CAD build for the part. Positions are in the model's coordinates, mm. A direction names the side the tool comes from. Round coordinates to 2 decimals unless told otherwise and drop trailing zeros. Order: outer loops, then holes, each group sorted by start corner. A loop starts at its lowest first (then second) coordinate and runs counter-clockwise, first axis right, second up. Notation, with made-up numbers: (31.25, 2.25) - (84.25, 2.25) arc R10 cw to (84.25, 6.25) - close; hole circle Ø11 at (23.25, 88.25). An arc over 180 degrees is marked (long way). Write item = value, one per line.
from build123d import *

# Parameters (mm, degrees)
CYLINDER291_R     = 2
CYLINDER291_DEPTH = 10
CYLINDER290_R     = 2
CYLINDER290_DEPTH = 10
BOX400_W          = 33
BOX400_H          = 22
BOX400_DEPTH      = 5
BOX397_W          = 33
BOX397_H          = 4
BOX397_DEPTH      = 20


with BuildPart() as cylinder291:
    # Cylinder291 → Cylinder291 (new body)
    with BuildSketch(Plane(origin=(-15, 72, 32), x_dir=(1, 0, 0), z_dir=(0, 0, 1))):
        Circle(CYLINDER291_R)
    extrude(amount=CYLINDER291_DEPTH)


with BuildPart() as fusion229:
    # Cylinder290 → Cylinder290 (new body)
    with BuildSketch(Plane(origin=(-36, 72, 32), x_dir=(1, 0, 0), z_dir=(0, 0, 1))):
        Circle(CYLINDER290_R)
    extrude(amount=CYLINDER290_DEPTH)

    # Fusion229: union Cylinder291
    add(cylinder291.part)


with BuildPart() as cut277:
    # Box400 → Box400 (new body)
    with BuildSketch(Plane(origin=(-42, 59, 37), x_dir=(1, 0, 0), z_dir=(0, 0, 1))):
        with Locations((16.5, 11)):
            Rectangle(BOX400_W, BOX400_H)
    extrude(amount=BOX400_DEPTH)

    # Cut277: cut Fusion229
    add(fusion229.part, mode=Mode.SUBTRACT)


with BuildPart() as lipo_cover:
    # Box397 → Box397 (new body)
    with BuildSketch(Plane(origin=(-42, 59, 37), x_dir=(1, 0, 0), z_dir=(0, 0, 1))):
        with Locations((16.5, 2)):
            Rectangle(BOX397_W, BOX397_H)
    extrude(amount=BOX397_DEPTH)

    # Fusion231: union Cut277
    add(cut277.part)


solid = lipo_cover.part
(1) Probe line 1 along X through (y, z) = (72, 40.3); line 2 along Y through (x, z) = (-15, 40.25); line 3 along Z through (x, y) = (-23.5, 78). List the from-to ranges inside material, lowest first.
Solved:
line_1 = -42 to -38, -34 to -17, -13 to -9
line_2 = 59 to 70, 74 to 81
line_3 = 37 to 42
(2) Pull direction X, two halves, no side cores. Call faces 3 (the flat face through (-9, 65, 40)), 4 (the cylindrical face through (-36, 74, 39)), 5 (the flat face through (-26, 63, 49)), 6 (the cylindrical face through (-15, 74, 39)): released by +X, released by -X, zero draft, split by the parting line, or undercut.
Solved:
face_3 = released by +X
face_4 = undercut
face_5 = zero draft
face_6 = undercut
(3) Band-saw the part on A-A on x = -36. List the corners of the cut face in (y, z).
Solved:
outline = (59, 37) - (70, 37) - (70, 42) - (63, 42) - (63, 57) - (59, 57) - close; (74, 37) - (81, 37) - (81, 42) - (74, 42) - close
(4) Band-saw the part on C-C on x = -22. List the corners of the cut face in (y, z), plus the area to 3 significant figures.
Solved:
outline = (59, 37) - (81, 37) - (81, 42) - (63, 42) - (63, 57) - (59, 57) - close
area = 170 mm²
(5) Tool access for faces 1 (the flat face through (-26, 72, 42)), 2 (the flat face through (-26, 61, 57)): list every direction of +Z, -Z, +X, -X, +Y, -Y with a clear straight run to the whole face (end or side of a thin tool).
Solved:
face_1 = +Z, +X, -X, +Y
face_2 = +Z, +X, -X, +Y, -Y
(6) Band-saw the part on D-D on z = 51. List the corners of the cut face in (x, y), plus the area to 3 significant figures.
Solved:
outline = (-42, 59) - (-9, 59) - (-9, 63) - (-42, 63) - close
area = 132 mm²
(7) Drop flat-ended pins along their axis: pin 1 (1 mm diameter, centred on x = -21, y = 78.5, fed in from +Z); pin 2 (3 mm diameter, centred on x = -15, y = 72, fed in from +Z); pin 3 (2 mm diameter, centred on x = -30, z = 46, fed in from +Y). Give the stop position or say it passes through.
Solved:
pin_1 = 42
pin_2 = through
pin_3 = 63
(8) Band-saw the part on B-B on y = 72. List the corners of the cut face in (x, z), plus the area to 3 significant figures.
Solved:
outline = (-42, 37) - (-38, 37) - (-38, 42) - (-42, 42) - close; (-34, 37) - (-17, 37) - (-17, 42) - (-34, 42) - close; (-13, 37) - (-9, 37) - (-9, 42) - (-13, 42) - close
area = 125 mm²
